Verification items for the finished model (mm, model axes). A direction names the side the tool comes from. Give positions to 0.01 mm unless a question says otherwise; leave off trailing zeros. Write each loop counter-clockwise with the first axis right and the second up, starting at its lowest first coordinate (ties: lowest second). Pieces come first, ordered by that corner, then holes. Notation, with made-up numbers: (17.5, 58) -> (43.5, 58) arc R20 cw to (43.5, 73) -> close; hole circle Ø6 at (74.5, -21.75). An arc over 180 degrees is marked (long way). Use one line per item in the form item = value. Start each with the question number.
(1) Scan lines: L1, parallel to Y at x = 15, z = 4.55; L2, parallel to Y at x = 9.5, z = 8.5; L3, parallel to X at y = -10, z = 10.25. Record each from-to range of solid material in increasing order.
(2) Release check for a two-part mould opening along X. For faces 1 (the face through (-11.247, -0.247, 2.218)), 2 (the face through (-12, 0, 12)), 3 (the face through (4.7, 2.6, 9)) record: pulls with the +X half, pulls with the -X half, needs draft (parallel to the pull), parting line crosses it, or undercut.
(3) Section check C-C, the plane x = -23. Record the cut outline in (y, z).
(4) Section check D-D, the plane y = -13.5. Record the cut outline in (x, z).
(5) Section check A-A, the plane x = -15. Record the cut outline in (y, z).
(6) Set-up check for faces 4 (the face through (-30.3, 14.9, 3.3)), 5 (the face through (-24.79, -17.72, 4.63)), 6 (the face through (18, -13, 6)), 7 (the face through (11, -11.25, 2)): record each of +Z, -Z, +X, -X, +Y, -Y from which the full face is reachable in a straight line by a thin tool's end or side.
(7) Section check B-B, the plane z = 7. State how many separate pieces and enclosed holes the cut face has, plus the area to 3 significant figures.
(8) Depth check by flat-ended pin: pin 1 Ø12 at (x, y) = (-9.5, 8) entering from -Z; pin 2 Ø5.5 at (x, y) = (-16.5, 14.5) entering from +Z. Enter the tip coordinate at first touch or a pass-through.
from build123d import *

# Parameters (mm, degrees)
SKETCH_W        = 55
SKETCH_H        = 66
PAD_DEPTH       = 12
POCKET_DEPTH    = 6
SKETCH002_R     = 3.3
POCKET001_DEPTH = 6.001
SKETCH003_R     = 4
POCKET002_DEPTH = 55.001
POCKET003_DEPTH = 4.5
SKETCH005_R     = 3.3
POCKET004_DEPTH = 5.5
POCKET005_DEPTH = 5.5


with BuildPart() as part:
    # Sketch → Pad (new body)
    with BuildSketch(Plane.XY):
        with Locations((-5.5, 0)):
            Rectangle(SKETCH_W, SKETCH_H)
    extrude(amount=PAD_DEPTH)

    # Sketch001 → Pocket (cut)
    with BuildSketch(Plane.XY.offset(12)):
        Polygon((18.1, 9.630642), (21.2, 15), (18.1, 20.369358), (11.9, 20.369358), (8.8, 15), (11.9, 9.630642), align=None)
        Polygon((-11.9, -20.369358), (-8.8, -15), (-11.9, -9.630642), (-18.1, -9.630642), (-21.2, -15), (-18.1, -20.369358), align=None)
        Polygon((11.9, -9.630642), (8.8, -15), (11.9, -20.369358), (18.1, -20.369358), (21.2, -15), (18.1, -9.630642), align=None)
        Polygon((-8.8, 15), (-11.9, 20.369358), (-18.1, 20.369358), (-21.2, 15), (-18.1, 9.630642), (-11.9, 9.630642), align=None)
        Polygon((3.1, -5.369358), (6.2, 0), (3.1, 5.369358), (-3.1, 5.369358), (-6.2, 0), (-3.1, -5.369358), align=None)
    extrude(amount=-POCKET_DEPTH, mode=Mode.SUBTRACT)

    # Sketch002 → Pocket001 (cut, through all)
    with BuildSketch(Plane.XY.offset(6)):
        with Locations((-15, 15)):
            Circle(SKETCH002_R)
        with Locations((15, 15)):
            Circle(SKETCH002_R)
        Circle(SKETCH002_R)
        with Locations((15, -15)):
            Circle(SKETCH002_R)
        with Locations((-15, -15)):
            Circle(SKETCH002_R)
    extrude(amount=-POCKET001_DEPTH, mode=Mode.SUBTRACT)

    # Sketch003 → Pocket002 (cut, through all)
    with BuildSketch(Plane.YZ.offset(22)):
        with Locations((-28, 0)):
            Circle(SKETCH003_R)
        with Locations((28, 0)):
            Circle(SKETCH003_R)
    extrude(amount=-POCKET002_DEPTH, mode=Mode.SUBTRACT)

    # Sketch004 → Pocket003 (cut)
    with BuildSketch(Plane(origin=(0, 0, 0), x_dir=(1, 0, 0), z_dir=(0, 0, -1))):
        with BuildLine():
            ThreePointArc((0, 11.25), (-11.25, 0), (0, -11.25))
            Line((0, -11.25), (22, -11.25))
            Line((22, 11.25), (22, -11.25))
            Line((0, 11.25), (22, 11.25))
        make_face()
    extrude(amount=-POCKET003_DEPTH, mode=Mode.SUBTRACT)

    # Sketch005 → Pocket004 (cut)
    with BuildSketch(Plane(origin=(-33, 0, 0), x_dir=(0, -1, 0), z_dir=(-1, 0, 0))):
        with Locations((-15, 0)):
            Circle(SKETCH005_R)
        with Locations((15, 0)):
            Circle(SKETCH005_R)
    extrude(amount=-POCKET004_DEPTH, mode=Mode.SUBTRACT)

    # Sketch006 → Pocket005 (cut)
    with BuildSketch(Plane(origin=(-27.5, 0, 0), x_dir=(0, -1, 0), z_dir=(-1, 0, 0))):
        Polygon((-9.630642, 3.1), (-15, 6.2), (-20.369358, 3.1), (-20.369358, -3.1), (-15, -6.2), (-9.630642, -3.1), align=None)
        Polygon((20.369358, 3.1), (15, 6.2), (9.630642, 3.1), (9.630642, -3.1), (15, -6.2), (20.369358, -3.1), align=None)
    extrude(amount=-POCKET005_DEPTH, mode=Mode.SUBTRACT)


solid = part.part
Completed:
q1.L1 = -33 to -18.3, -11.7 to 11.7, 18.3 to 33
q1.L2 = -33 to -16.21, -13.79 to 13.79, 16.21 to 33
q1.L3 = -33 to -18.31, -11.69 to 11.69, 18.31 to 22
q2.face_1 = pulls with the +X half
q2.face_2 = needs draft
q2.face_3 = undercut
q3.outline = (-33, 0) -> (-32, 0) arc R4 cw to (-24, 0) -> (-20.37, 0) -> (-20.37, 3.1) -> (-15, 6.2) -> (-9.63, 3.1) -> (-9.63, 0) -> (9.63, 0) -> (9.63, 3.1) -> (15, 6.2) -> (20.37, 3.1) -> (20.37, 0) -> (24, 0) arc R4 cw to (32, 0) -> (33, 0) -> (33, 12) -> (-33, 12) -> close
q4.outline = (-33, 2.94) -> (-27.5, 2.94) -> (-27.5, 5.33) -> (-22, 5.33) -> (-22, 0) -> (-17.94, 0) -> (-17.94, 6) -> (-20.33, 6) -> (-20.33, 12) -> (-33, 12) -> close; (-12.06, 0) -> (12.06, 0) -> (12.06, 6) -> (9.67, 6) -> (9.67, 12) -> (-9.67, 12) -> (-9.67, 6) -> (-12.06, 6) -> close; (17.94, 0) -> (22, 0) -> (22, 12) -> (20.33, 12) -> (20.33, 6) -> (17.94, 6) -> close
q5.outline = (-33, 0) -> (-32, 0) arc R4 cw to (-24, 0) -> (-18.3, 0) -> (-18.3, 6) -> (-20.37, 6) -> (-20.37, 12) -> (-33, 12) -> close; (-11.7, 0) -> (11.7, 0) -> (11.7, 6) -> (9.63, 6) -> (9.63, 12) -> (-9.63, 12) -> (-9.63, 6) -> (-11.7, 6) -> close; (18.3, 0) -> (24, 0) arc R4 cw to (32, 0) -> (33, 0) -> (33, 12) -> (20.37, 12) -> (20.37, 6) -> (18.3, 6) -> close
q6.face_4 = -Z, -X
q6.face_5 = -Z
q6.face_6 = +Z
q6.face_7 = -Z, +X
q7.separate_pieces = 1
q7.enclosed_holes = 5
q7.area = 3,130 mm²
q8.pin_1 = 0
q8.pin_2 = 6
